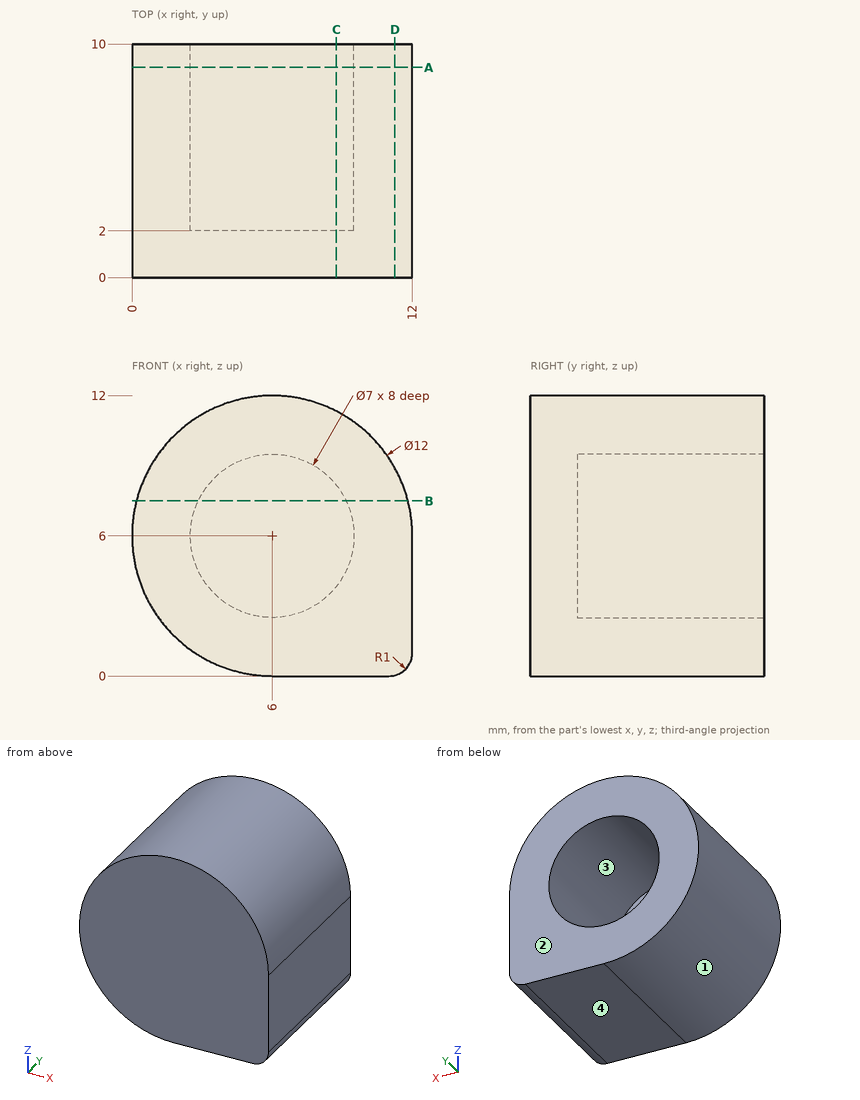
Study the drawing (mm; zero at the part's minimum x, y, z) and answer. Round coordinates to 2 decimals unless told otherwise and drop trailing zeros. Write each loop counter-clockwise with the first axis right and the second up, starting at its lowest first coordinate (ties: lowest second). Pieces come first, ordered by that corner, then holes. Notation, with made-up numbers: (1, -20.75) - (32, -20.75) arc R21 cw to (32, -15.75) - close; hole circle Ø7 at (-14, 26.5). An arc over 180 degrees is marked (long way). Return JSON: item names as keys, results as strings. Group by question number.
Q1. The part is cut by section A-A on y = 9. Write down the section's boundary in (x, z), then the cut area to 3 significant figures.
Q2. The mould has two halves that part along Z. Classify the marked faces 1, 2, 3 and 4: released by +Z, released by -Z, zero draft, split by the parting line, or undercut.
Q3. The part is cut by section D-D on x = 11.25. Write down the section's boundary in (y, z), then the cut area to 3 significant figures.
Q4. The part is cut by section B-B on z = 7.5. Write down the section's boundary in (x, y), then the cut area to 3 significant figures.
Q5. This flat-tipped pin is pushed along its axis until it touches: pin 1 Ø4 at (x, y) = (2.5, 1.5) entering from -Z. Where does it stop, or does it pass through?
Q6. Find the intervals of material crossed by L1, parallel to X at y = 4.5, z = 6; L2, parallel to Y at x = 5, z = 5.75, in increasing order.
Q7. The part is cut by section C-C on x = 8.75. Write down the section's boundary in (y, z), then the cut area to 3 significant figures.
Solved:
{
 "1": {"outline": "(6, 0) - (11, 0) arc R1 ccw to (12, 1) - (12, 6) arc R6 ccw (long way) to start; hole circle Ø7 at (6, 6)", "area": "82.1 mm²"},
 "2": {"face 1": "split by the parting line", "face 2": "zero draft", "face 3": "undercut", "face 4": "released by -Z"},
 "3": {"outline": "(0, 0.03) - (10, 0.03) - (10, 8.9) - (0, 8.9) - close", "area": "88.7 mm²"},
 "4": {"outline": "(0.19, 0) - (11.81, 0) - (11.81, 10) - (9.16, 10) - (9.16, 2) - (2.84, 2) - (2.84, 10) - (0.19, 10) - close", "area": "65.6 mm²"},
 "5": {"pin 1": "z = 0.19"},
 "6": {"L1": "0 to 2.5, 9.5 to 12", "L2": "0 to 2"},
 "7": {"outline": "(0, 0) - (10, 0) - (10, 3.83) - (2, 3.83) - (2, 8.17) - (10, 8.17) - (10, 11.33) - (0, 11.33) - close", "area": "78.7 mm²"}
}
